Build history of the part. All positions in model axes, mm. A direction names the side the tool comes from. Coordinates: 2 decimals unless noted, no trailing zeros. Order: outer loops, then holes, each group sorted by start corner. A loop starts at its lowest first (then second) coordinate and runs counter-clockwise, first axis right, second up. Notation, with made-up numbers: (39.25, 69) - (65.25, 69) arc R20 cw to (65.25, 88) - close; hole circle Ø8 at (-22, -40). An arc over 180 degrees is marked (long way). Return JSON: item names as keys, results as strings.
from build123d import *

# Parameters (mm, degrees)
SKETCH_1_R          = 4.75
EXTRUDE_1_DEPTH     = 1.4
SKETCH_2_R          = 1.5
EXTRUDE_2_DEPTH     = 4
SKETCH_3_W          = 0.760348124
SKETCH_3_H          = 2.271623197
SKETCH_3_W_2        = 1.135811598
SKETCH_3_H_2        = 0.62458345
CUT_EXTRUDE_1_DEPTH = 1


with BuildPart() as part:
    # 草图1 → 凸台-拉伸1 (new body)
    with BuildSketch(Plane.XY):
        Circle(SKETCH_1_R)
    extrude(amount=EXTRUDE_1_DEPTH)

    # 草图2 → 凸台-拉伸2 (add)
    with BuildSketch(Plane.XY.offset(1.4)):
        Circle(SKETCH_2_R)
    extrude(amount=EXTRUDE_2_DEPTH)

    # 草图3 → 切除-拉伸1 (cut)
    with BuildSketch(Plane(origin=(0, 0, 0), x_dir=(-1, 0, 0), z_dir=(0, 0, -1))):
        with Locations((0, 1.448103324)):
            Rectangle(SKETCH_3_W, SKETCH_3_H)
        with Locations((-0.948079861, 0)):
            Rectangle(SKETCH_3_W_2, SKETCH_3_H_2)
        with Locations((0.948079861, 0)):
            Rectangle(SKETCH_3_W_2, SKETCH_3_H_2)
        with Locations((0, -1.448103324)):
            Rectangle(SKETCH_3_W, SKETCH_3_H)
        Rectangle(SKETCH_3_W, SKETCH_3_H_2)
    extrude(amount=-CUT_EXTRUDE_1_DEPTH, mode=Mode.SUBTRACT)


solid = part.part
1. Cut at A-A on z = 0.65. Give the cut face in (x, y).
Check values:
{"outline": "circle Ø9.5 at (0, 0); hole (-1.52, -0.31) - (-0.38, -0.31) - (-0.38, -2.58) - (0.38, -2.58) - (0.38, -0.31) - (1.52, -0.31) - (1.52, 0.31) - (0.38, 0.31) - (0.38, 2.58) - (-0.38, 2.58) - (-0.38, 0.31) - (-1.52, 0.31) - close"}
2. Cut at C-C on x = 0. Give the cut face in (y, z).
Check values:
{"outline": "(-4.75, 0) - (-2.58, 0) - (-2.58, 1) - (2.58, 1) - (2.58, 0) - (4.75, 0) - (4.75, 1.4) - (1.5, 1.4) - (1.5, 5.4) - (-1.5, 5.4) - (-1.5, 1.4) - (-4.75, 1.4) - close"}
3. Drop flat-ended pins along their axis: pin 1 (1.1 mm diameter, centred on y = 2, z = 0.5, fed in from -X); pin 2 (1.1 mm diameter, centred on x = 1, z = 0.5, fed in from +Y); pin 3 (3 mm diameter, centred on x = 2.5, y = -1, fed in from -Z); pin 4 (0.5 mm diameter, centred on y = 2, z = 0.5, fed in from +X). Give the stop position or say it passes through.
Check values:
{"pin 1": "x = -4.52", "pin 2": "y = 4.73", "pin 3": "z = 0", "pin 4": "x = 4.42"}
4. Tool access for faces 1 (the flat face through (1, -1, 0)), 2 (the cylindrical face through (-1.5, 0.07, 3.37)), 3 (the flat face through (1, 0.312, 0.5)): list every direction of +Z, -Z, +X, -X, +Y, -Y with a clear straight run to the whole face (end or side of a thin tool).
Check values:
{"face 1": "-Z, +X, -X, +Y, -Y", "face 2": "+Z", "face 3": "-Z"}
5. Cut at B-B on y = 0. Give the cut face in (x, z).
Check values:
{"outline": "(-4.75, 0) - (-1.52, 0) - (-1.52, 1) - (1.52, 1) - (1.52, 0) - (4.75, 0) - (4.75, 1.4) - (1.5, 1.4) - (1.5, 5.4) - (-1.5, 5.4) - (-1.5, 1.4) - (-4.75, 1.4) - close"}
6. Cut at D-D on z = 3.25. Give the cut face in (x, y), plus the area to 3 significant figures.
Check values:
{"outline": "circle Ø3 at (0, 0)", "area": "7.07 mm²"}
7. Probe L1, parallel to Z at x = -0.75, y = -1.5; L2, parallel to X at y = 0.75, z = 0.85; L3, parallel to X at y = 1.5, z = 0.45. List the from-to ranges inside material, lowest first.
Check values:
{"L1": "0 to 1.4", "L2": "-4.69 to -0.38, 0.38 to 4.69", "L3": "-4.51 to -0.38, 0.38 to 4.51"}
8. Mould opens along X. For faces 4 (the cylindrical face through (2.192, -4.214, 0.69)), 5 (the flat face through (0, 0, 5.4)), 6 (the flat face through (0.38, -1.5, 0.5)) say: pulls with the +X half, pulls with the -X half, needs draft (parallel to the pull), parting line crosses it, or undercut.
Check values:
{"face 4": "parting line crosses it", "face 5": "needs draft", "face 6": "undercut"}
